```python
from build123d import *

# Parameters (mm, degrees)
BOSS_EXTRUDE1_DEPTH = 10
FILLET4_R           = 1
CIRPATTERN1_COUNT   = 18


with BuildPart() as part:
    # Sketch1 → Boss-Extrude1 (new body)
    with BuildSketch(Plane(origin=(0, 0, 0), x_dir=(1, 0, 0), z_dir=(0, 1, 0))):
        with BuildLine():
            ThreePointArc((38.602544551, -3.377285031), (38.418488378, -5.057889949), (38.161300429, -6.728866885))
            Line((38.161300429, -6.728866885), (0, 0))
            Line((0, 0), (38.161300429, 6.728866885))
            ThreePointArc((38.161300429, 6.728866885), (38.418488378, 5.057889949), (38.602544551, 3.377285031))
            Line((38.602544551, 3.377285031), (42.124092809, 3.685380582))
            ThreePointArc((42.124092809, 3.685380582), (46.141395468, 3.478911596), (49.948794335, 2.180811458))
            ThreePointArc((49.948794335, 2.180811458), (49.99637981, 0), (49.948794335, -2.180811458))
            ThreePointArc((49.948794335, -2.180811458), (46.141395468, -3.478911596), (42.124092809, -3.685380582))
            Line((42.124092809, -3.685380582), (38.602544551, -3.377285031))
        make_face()
    boss_extrude1 = extrude(amount=BOSS_EXTRUDE1_DEPTH)

    # Fillet4
    fillet4_edges = [part.edges().sort_by_distance(p)[0] for p in [
        (38.602544551, 5, 3.377285031),
    ]]
    fillet(fillet4_edges, radius=FILLET4_R)

    # CirPattern1: Boss-Extrude1 ×18 about axis
    cirpattern1_axis = Axis((0, 0, 0), (0, 1, 0))
    for i in range(1, CIRPATTERN1_COUNT):
        add(boss_extrude1.rotate(cirpattern1_axis, i * 360 / CIRPATTERN1_COUNT))


solid = part.part
```
Could you check a few things on this model? Use its own coordinates, in mm. A direction names the side the tool comes from. Coordinates: 2 decimals unless noted, no trailing zeros. Order: outer loops, then holes, each group sorted by start corner. A loop starts at its lowest first (then second) coordinate and runs counter-clockwise, first axis right, second up. Notation, with made-up numbers: M -26.75,78.5 L -13.75,78.5 A11 cw -13.75,98.5 Z; hole C -6.75,-27.5 d2. An arc over 180 degrees is marked long. Use one line per item in the form item = value. Start each with the question number.
1. We'd pull the mould along X, two halves only. Please class faces 4 (the cylindrical face through (25.025, 4.93, 43.283)), 5 (the cylindrical face through (-33.16, 4.93, -32.35)), 6 (the flat face through (36.74, 4.93, 17.13)), 7 (the flat face through (-39.11, 4.93, -10.48)): +X half, -X half, draft (parallel to the pull), parting line (faces both ways), or undercut.
2. Suppose I cut it at A-A on x = 14.5. Write out the boundary of the cut face in (y, z).
3. Suppose I cut it at B-B on x = -15. Write out the boundary of the cut face in (y, z).
4. For pin 1 (2 mm diameter, centred on x = -4.5, y = 6.5, fed in from +Z); pin 2 (3 mm diameter, centred on y = 8, z = 25.5, fed in from -X); pin 3 (3 mm diameter, centred on x = 27, y = 1.5, fed in from -Z), each with a flat end and sliding along its axis, tell me the tip position at first contact or that it passes through.
5. Please list where these lines run through material, in increasing order: line 1 (X direction, y = 0.5, z = 41) (3 decimals); line 2 (Z direction, x = 35, y = 7.5); line 3 (Z direction, x = 39, y = 2).
6. On a 3-axis mill with a long thin cutter (end or side, diameter ignored), from which of +Z, -Z, +X, -X, +Y, -Y can I reach the whole of each face in a straight line? I mean faces 1 (the cylindrical face through (-33.061, 4.93, 32.297)), 2 (the flat face through (-29, 5, -29)), 3 (the cylindrical face through (-37.547, 4.93, -26.95)). Say none if no direction works.
Geometry says:
q1.face_4 = +X half
q1.face_5 = undercut
q1.face_6 = undercut
q1.face_7 = -X half
q2.outline = M 0,-35.93 L 10,-35.93 L 10,35.93 L 0,35.93 Z
q3.outline = M 0,-35.73 L 10,-35.73 L 10,35.73 L 0,35.73 Z
q4.pin_1 = 47.99
q4.pin_2 = -37.59
q4.pin_3 = -43
q5.line_1 = -26.75 to -19.49, -10.985 to -3.587, 3.587 to 10.985, 19.49 to 26.75
q5.line_2 = -33.21 to -24.52, -16.63 to 16.63, 24.52 to 33.21
q5.line_3 = -31.28 to -29.08, -18.17 to -10.45, -3.41 to 3.59, 10.45 to 18.17, 29.08 to 31.28
q6.face_1 = +Z, +Y, -Y
q6.face_2 = -Z, +Y, -Y
q6.face_3 = -X, +Y, -Y
